Check sheet for the modelled part. Datum: model origin and axes. Units: mm. A direction names the side the tool comes from. Give positions to 0.01 mm unless a question says otherwise; leave off trailing zeros. Write each loop counter-clockwise with the first axis right and the second up, starting at its lowest first coordinate (ties: lowest second). Pieces come first, ordered by that corner, then holes. Notation, with made-up numbers: (14, 80.25) -> (64, 80.25) arc R29 cw to (64, 113.25) -> close; hole circle Ø10 at (30, 37). An arc over 180 degrees is marked (long way). Use a Markdown table: item, result. Add a question column.
1. Cross-section at C-C (z = -9.5). Enter the section's corners in (x, y), then the cut area to 3 significant figures.
2. Cross-section at A-A (x = 0). Enter the section's corners in (y, z), then the cut area to 3 significant figures.
3. Cross-section at D-D (z = -141). Enter the section's corners in (x, y).
4. Gauge pin test, flat ends, axial feed: P1, Ø1.5, axis at y = -3.5, z = -128, coming from the -X side; P2, Ø3, axis at y = -2.5, z = -109.5, coming from the +X side; P3, Ø3, axis at x = 4, z = 36.5, coming from the -Y side; P4, Ø6, axis at x = -3.5, y = -4, coming from the -Z side. Record the tip position at first contact, or that the pin passes through.
5. Scan lines: probe 1 along Z at (x, y) = (-4.5, 1.75); probe 2 along X at (y, z) = (-0.75, 114.5); probe 3 along X at (y, z) = (-1, -49). Record each from-to range of solid material in increasing order. Write a range as [from, to].
6. Set-up check for faces 1 (the cylindrical face through (-7.493, 0.33, 1.554)), 2 (the cylindrical face through (-0.59, 4.46, 142.41)), 3 (the flat face through (-5, 0, -113)): record each of +Z, -Z, +X, -X, +Y, -Y from which the full face is reachable in a straight line by a thin tool's end or side.
from build123d import *

# Parameters (mm, degrees)
SKETCH_1_R      = 4.5
EXTRUDE_1_DEPTH = 173
EXTRUDE_START   = -60
SKETCH_2_R      = 7.5
EXTRUDE_2_DEPTH = 226
CHAMFER_1_SIZE  = 2


with BuildPart() as part:
    # 草图1 → 凸台-拉伸1 (new, symmetric)
    with BuildSketch(Plane.XY):
        Circle(SKETCH_1_R)
    extrude(amount=EXTRUDE_1_DEPTH, both=True)

    # 草图2 → 凸台-拉伸2 (add)
    with BuildSketch(Plane.XY.offset(173).offset(EXTRUDE_START)):
        Circle(SKETCH_2_R)
    extrude(amount=-EXTRUDE_2_DEPTH)

    # 倒角1
    chamfer_1_edges = [part.edges().sort_by_distance(p)[0] for p in [
        (-4.5, 0, -173),
        (-4.5, 0, 173),
        (-7.5, 0, 113),
        (-7.5, 0, -113),
    ]]
    chamfer(chamfer_1_edges, length=CHAMFER_1_SIZE)


solid = part.part
Worked answers:
| question | item | result |
|---|---|---|
| 1 | outline | circle Ø15 at (0, 0) |
| 1 | area | 177 mm² |
| 2 | outline | (-7.5, -111) -> (-5.5, -113) -> (-4.5, -113) -> (-4.5, -171) -> (-2.5, -173) -> (2.5, -173) -> (4.5, -171) -> (4.5, -113) -> (5.5, -113) -> (7.5, -111) -> (7.5, 111) -> (5.5, 113) -> (4.5, 113) -> (4.5, 171) -> (2.5, 173) -> (-2.5, 173) -> (-4.5, 171) -> (-4.5, 113) -> (-5.5, 113) -> (-7.5, 111) -> close |
| 2 | area | 4,450 mm² |
| 3 | outline | circle Ø9 at (0, 0) |
| 4 | P1 | stops at x = -3.56 |
| 4 | P2 | stops at x = 7.43 |
| 4 | P3 | stops at y = -7.07 |
| 4 | P4 | stops at z = -173 |
| 5 | probe 1 | z = [-113, 113] |
| 5 | probe 2 | x = [-4.44, 4.44] |
| 5 | probe 3 | x = [-7.43, 7.43] |
| 6 | face 1 | +Z, -Z |
| 6 | face 2 | +Z |
| 6 | face 3 | -Z |
